The model under review builds one solid part; all positions refer to its coordinate system, in mm. A direction names the side the tool comes from. Coordinates: 2 decimals unless noted, no trailing zeros. Write each loop counter-clockwise with the first axis right and the second up, starting at its lowest first coordinate (ties: lowest second). Pieces come first, ordered by that corner, then holes. Notation, with made-up numbers: (31.25, -33.75) -> (75.25, -33.75) arc R5 cw to (75.25, -28.75) -> close; hole circle Ø2 at (83, 83.25). An arc over 180 degrees is marked (long way). Write each question's results on one line, items separated by ' | '.
```python
from build123d import *

# Parameters (mm, degrees)
F6_W    = 40
F6_H    = 40
F6_W_2  = 36
F6_H_2  = 36
F5_W    = 40
F5_H    = 40
F5_W_2  = 36
F5_H_2  = 36
F13_W   = 40
F13_H   = 40
F13_W_2 = 36
F13_H_2 = 36
F20_W   = 40
F20_H   = 40
F20_W_2 = 36
F20_H_2 = 36
F25_W   = 40
F25_H   = 40
F25_W_2 = 36
F25_H_2 = 36


with BuildPart() as f11:
    # F11: sweep along a path in F2, F7, F10
    with BuildLine(Plane(origin=(0, 0, 0), x_dir=(1, 0, 0), z_dir=(0, -0.3583679495, 0.9335804265))) as f11_path:
        Line((0, 0), (764.0288873983, 496.1661608987))
    with BuildLine(Plane.XY) as f11_path_2:
        Line((0, 0), (-229, -800))
    with BuildLine(Plane(origin=(0, -102.742069809, -267.6522425435), x_dir=(1, 0, 0), z_dir=(0, -0.3583679495, -0.9335804265))) as f11_path_3:
        Line((-950.6889298291, 1197.8256350602), (-229, 746.8643411978))
    # F6 (on line) → F11 (sweep)
    with BuildSketch(Plane(origin=(764.0288873983, 463.2110161053, 177.810049715), x_dir=(-0.4952299095, 0.8610830461, -0.1152533056), z_dir=(0.8386705679, 0.5084643426, 0.1951811742))):
        Rectangle(F6_W, F6_H)
        Rectangle(F6_W_2, F6_H_2, mode=Mode.SUBTRACT)
    sweep(path=f11_path.line + f11_path_2.line + f11_path_3.line, transition=Transition.RIGHT)

    # F14: sweep along a path in F2
    with BuildLine(Plane(origin=(0, 0, 0), x_dir=(1, 0, 0), z_dir=(0, -0.3583679495, 0.9335804265))) as f14_path:
        Line((0, 0), (-514.7840798788, 635.7053964718))
    # F5 (on line) → F14 (sweep)
    with BuildSketch(Plane(origin=(-514.7840798788, 593.4821151647, 227.8164394485), x_dir=(-0.7771459615, -0.5875211991, -0.2255282581), z_dir=(-0.629320391, 0.7255282581, 0.2785042047))):
        Rectangle(F5_W, F5_H)
        Rectangle(F5_W_2, F5_H_2, mode=Mode.SUBTRACT)
    sweep(path=f14_path.line)

    # F15: sweep along a path in F10
    with BuildLine(Plane(origin=(0, -102.742069809, -267.6522425435), x_dir=(1, 0, 0), z_dir=(0, -0.3583679495, -0.9335804265))) as f15_path:
        Line((-229, 746.8643411978), (271.5327794398, 1387.51708388))
    # F13 (on line) → F15 (sweep)
    with BuildSketch(Plane(origin=(776.072475672, -927.3510842252, 355.9767290852), x_dir=(0.7880107536, 0.5747695027, -0.2206333405), z_dir=(0.6156614753, -0.7356714154, 0.282397798))):
        with Locations((-640.2700647459, -286.6943596362)):
            Rectangle(F13_W, F13_H)
        with Locations((-640.2700647459, -286.6943596362)):
            Rectangle(F13_W_2, F13_H_2, mode=Mode.SUBTRACT)
    sweep(path=f15_path.line)

    # F21: sweep along a path in F18
    with BuildLine(Plane(origin=(0, -289.7450576732, 384.5046783753), x_dir=(1, 0, 0), z_dir=(0, 0.6018150232, -0.79863551))) as f21_path:
        Line((-229, 638.9084080378), (112.5, 1230.4037588226))
    # F20 (on line) → F21 (sweep)
    with BuildSketch(Plane(origin=(560.9054560261, -775.8877736222, -584.6733742383), x_dir=(0.8660254038, 0.399317755, 0.3009075116), z_dir=(0.5, -0.6916386401, -0.5211870984))):
        with Locations((-517.7740214856, 481.4520185216)):
            Rectangle(F20_W, F20_H)
        with Locations((-517.7740214856, 481.4520185216)):
            Rectangle(F20_W_2, F20_H_2, mode=Mode.SUBTRACT)
    sweep(path=f21_path.line)

    # F26: sweep along a path in F23
    with BuildLine(Plane(origin=(290.0513412295, -497.2032011274, 0), x_dir=(-0.8637666966, -0.5038919466, 0), z_dir=(-0.5038919466, 0.8637666966, 0))) as f26_path:
        Line((1108.6913477208, 98.2169269961), (1182.3538043363, -506.3116848044))
    # F25 (on line) → F26 (sweep)
    with BuildSketch(Plane(origin=(-67.4518628313, -39.3491096563, -640.8673626896), x_dir=(0.9945271851, -0.006402875, -0.1042817402), z_dir=(-0.1044781228, -0.0609489633, -0.992657819))):
        with Locations((-667.4273420568, 1059.8983464665)):
            Rectangle(F25_W, F25_H)
        with Locations((-667.4273420568, 1059.8983464665)):
            Rectangle(F25_W_2, F25_H_2, mode=Mode.SUBTRACT)
    sweep(path=f26_path.line)


solid = f11.part
```
Q1. Add section C-C (z = -243.5). Write out the cut boundary in (x, y).
Solution:
outline: (-723.8, -1096.88) -> (-683.58, -1096.88) -> (-683.33, -1056.81) -> (-723.55, -1056.81) -> close; (-33.82, -1089.9) -> (-3.17, -1156.37) -> (43.02, -1156.37) -> (12.37, -1089.9) -> close; hole (-721.78, -1094.88) -> (-685.58, -1094.88) -> (-685.35, -1058.81) -> (-721.55, -1058.81) -> close; hole (-29.97, -1093.23) -> (-2.39, -1153.04) -> (39.18, -1153.04) -> (11.59, -1093.23) -> close
Q2. Add section B-B (y = 231.5). Write out the cut boundary in (x, z), plus the area to 3 significant figures.
Solution:
outline: (-232.75, 110.29) -> (-220.32, 67.44) -> (-168.85, 67.44) -> (-181.28, 110.29) -> close; (339, 99.43) -> (348.06, 60.47) -> (424.68, 78.3) -> (415.62, 117.26) -> close; hole (-229.56, 108.15) -> (-218.37, 69.58) -> (-172.05, 69.58) -> (-183.24, 108.15) -> close; hole (343.28, 98.37) -> (351.44, 63.31) -> (420.4, 79.36) -> (412.24, 114.42) -> close | area: 1,020 mm²
Q3. Clearance check with a flat-ended pin moving along its axis: P1, Ø8, axis at y = -988.5, z = 63, coming from the +X side. State where the tip first meets the part, or that it passes through.
Solution:
P1: x = -45.36
Q4. Draft analysis for pull direction Z (two halves, no side actions). For faces 5 (the flat face through (-246.16, 313.36, 120.59)), 6 (the flat face through (-96.14, -400.21, 3.24)), 7 (the flat face through (388.41, 232.41, 69.86)), state which applies: pulls with the +Z half, pulls with the -Z half, needs draft (parallel to the pull), parting line crosses it, or undercut.
Solution:
face 5: pulls with the +Z half | face 6: undercut | face 7: pulls with the -Z half
Q5. Add section D-D (z = -403.5). Write out the cut boundary in (x, y).
Solution:
outline: (-740.64, -1106.71) -> (-700.42, -1106.71) -> (-700.17, -1066.63) -> (-740.39, -1066.63) -> close; hole (-738.62, -1104.7) -> (-702.42, -1104.7) -> (-702.19, -1068.64) -> (-738.39, -1068.64) -> close
Q6. For line 1 (X direction, y = 389.5, z = 158.5); line 2 (Y direction, x = 565.5, z = 111.5); line 3 (Z direction, x = -497.5, y = -969.5), list the stretches that pass through material, from the lowest coordinate up. Write a range as from..to.
Solution:
line 1: -366.19..-363.62, -317.3..-314.72, 599.97..604.01, 676.7..680.74 | line 2: 316.93..363.38 | line 3: 43.39..45.5, 83.57..85.68
Q7. Machinability: for faces 1 (the flat face through (-261.658, 309.242, 97.284)), 2 (the flat face through (373.896, 249.872, 86.728)), 3 (the flat face through (-117.383, -394.992, 19.567)), 4 (the flat face through (-70.71, -1047.56, -186.86)), which of the approach directions +Z, -Z, +X, -X, +Y, -Y give a long, thin tool a straight path to every point of the face, cutting with its end or side? Answer none if there is none.
Solution:
face 1: -Z, -X, +Y | face 2: -Z, +Y | face 3: +Z, -X | face 4: none
Q8. Add section A-A (x = 67). Write out the cut boundary in (y, z), plus the area to 3 significant figures.
Solution:
outline: (-1253.43, -316.64) -> (-1229.36, -348.59) -> (-1165.47, -300.44) -> (-1189.54, -268.5) -> close; (-1191.19, 128.74) -> (-1130.54, 105.46) -> (-1116.2, 142.8) -> (-1176.86, 166.09) -> close; (14.65, -4.94) -> (61.1, -4.94) -> (66.6, 36.13) -> (20.14, 36.13) -> close; hole (-1249.03, -315.83) -> (-1227.37, -344.58) -> (-1169.87, -301.25) -> (-1191.53, -272.5) -> close; hole (-1187.44, 129.45) -> (-1132.85, 108.49) -> (-1119.95, 142.1) -> (-1174.54, 163.05) -> close; hole (17.24, -2.89) -> (59.05, -2.89) -> (64, 34.07) -> (22.19, 34.07) -> close | area: 1,460 mm²
